For this review, take the finished solid that the model builds, in its own axes (mm). A direction names the side the tool comes from. Round coordinates to 2 decimals unless told otherwise and drop trailing zeros. Loops run counter-clockwise (first coordinate to the right, second up) from the corner with the lowest first, then second, coordinate; pieces in that order, holes last. Notation, with made-up numbers: M 36,-12 L 60,-12 A15 cw 60,8 Z; hole C -26,82.25 d5. An arc over 180 degrees is marked long. One line per question, with ' | ' between items. Start each with the question number.
1) Mouldability with a two-part tool opening along Z and no side actions: class faces 1 (the face through (-2.57, 0.8, -0.28)), 2 (the face through (4, 1, 0)), 3 (the face through (-1, 0, 1)) as pulls with the +Z half, pulls with the -Z half, needs draft (parallel to the pull), parting line crosses it, or undercut.
2) For probe 1 along X at (y, z) = (1.45, 1.75); probe 2 along X at (y, z) = (3.85, 4.5); probe 3 along Y at (x, z) = (-4.25, -5.5), list the stretches that pass through material, from the lowest coordinate up. Write a range as from..to.
3) For pin 1 Ø0.9 at (x, z) = (3.5, 3.5) entering from -Y; pin 2 Ø4 at (x, z) = (3, 6) entering from -Y; pin 3 Ø1 at (x, z) = (-3.97, 3.97) entering from -Y; pin 4 Ø0.9 at (x, y) = (3.5, 2) entering from -Z, all flat-tipped, find the tip position at first contact; note any pin that passes through.
4) For faces 4 (the face through (4.49, 2.53, 4.64)), 5 (the face through (-4, 1, -7.938)), 6 (the face through (3.862, 4.114, 6.405)), list the 3-axis set-ups (+Z, -Z, +X, -X, +Y, -Y) from which the entire face can be reached by the end or side of a thin tool; tool diameter is ignored.
5) We need section C-C (y = 3.9). Give the boundary of the cut face in (x, z).
```python
from build123d import *

# Parameters (mm, degrees)
SKETCH1_W               = 15.875
SKETCH1_H               = 15.875
BASE_EXTRUDE_DEPTH      = 3.175
SKETCH2_R               = 2.4384
BOSS_EXTRUDE1_DEPTH     = 1.905
LPATTERN4_COUNT         = 2
LPATTERN4_PITCH         = 7.9375
LPATTERN4_COUNT_DIR2    = 2
LPATTERN4_PITCH_DIR2    = 7.9375
CUT_EXTRUDE1_DEPTH      = 7.9375
CUT_EXTRUDE1_DEPTH_BACK = 12.6656949
SHELL1_T                = -1.5875
SKETCH4_R               = 1.27
BOSS_EXTRUDE2_DEPTH     = 1.5875
CUT_EXTRUDE2_START      = -1.5875
SKETCH5_R               = 0.635
CUT_EXTRUDE2_DEPTH      = 1.5875
FILLET1_R               = 0.254


with BuildPart() as part:
    # Sketch1 → Base-Extrude (new body)
    with BuildSketch(Plane(origin=(0, 0, 0), x_dir=(1, 0, 0), z_dir=(0, 1, 0))):
        Rectangle(SKETCH1_W, SKETCH1_H)
    extrude(amount=BASE_EXTRUDE_DEPTH)

    # Sketch2 → Boss-Extrude1 (add)
    with BuildSketch(Plane(origin=(0, 3.175, 0), x_dir=(-1, 0, 0), z_dir=(0, 1, 0))):
        with Locations(Location((3.96875, 3.96875, 0), (0, 0, 270))):
            Circle(SKETCH2_R)
    boss_extrude1 = extrude(amount=BOSS_EXTRUDE1_DEPTH)

    # LPattern4: Boss-Extrude1 2 × 2
    with Locations(*[(i * LPATTERN4_PITCH, 0, -j * LPATTERN4_PITCH_DIR2) for i in range(LPATTERN4_COUNT) for j in range(LPATTERN4_COUNT_DIR2) if (i, j) != (0, 0)]):
        add(boss_extrude1)

    # Sketch3 → Cut-Extrude1 (cut, two sides: drawn at the far end of the back side and taken through both)
    with BuildSketch(Plane(origin=(0, 3.175, 0), x_dir=(-1, 0, 0), z_dir=(0, 1, 0)).offset(-CUT_EXTRUDE1_DEPTH_BACK)):
        Polygon((0, -53.435079143), (0, -7.9375), (0, 0), (-7.9375, 0), (-53.435079143, 0), (-117.778372622, -64.343293479), (-64.343293479, -117.778372622), align=None)
    extrude(amount=CUT_EXTRUDE1_DEPTH + CUT_EXTRUDE1_DEPTH_BACK, mode=Mode.SUBTRACT)

    # Shell1
    shell1_openings = [part.faces().sort_by_distance(p)[0] for p in [
        (-1.322916667, 0, 1.322916667),
    ]]
    offset(amount=SHELL1_T, openings=shell1_openings, kind=Kind.INTERSECTION)

    # Sketch4 → Boss-Extrude2 (add)
    with BuildSketch(Plane.XZ.offset(-1.5875)):
        with Locations(Location((-3.81, 0, 0), (0, 0, 90))):
            Circle(SKETCH4_R)
        with Locations(Location((0, 3.81, 0), (0, 0, 90))):
            Circle(SKETCH4_R)
    extrude(amount=BOSS_EXTRUDE2_DEPTH)

    # Sketch5 → Cut-Extrude2 (cut)
    with BuildSketch(Plane.XZ.offset(CUT_EXTRUDE2_START)):
        with Locations(Location((0, 3.81, 0), (0, 0, 270))):
            Circle(SKETCH5_R)
        with Locations(Location((-3.81, 0, 0), (0, 0, 270))):
            Circle(SKETCH5_R)
    extrude(amount=CUT_EXTRUDE2_DEPTH, mode=Mode.SUBTRACT)

    # Fillet1
    fillet1_edges = [part.edges().sort_by_distance(p)[0] for p in [
        (7.9375, 3.175, 3.96875),
        (-3.96875, 3.175, -7.9375),
        (0, 3.175, -3.96875),
        (3.96875, 3.175, 0),
        (-7.9375, 3.175, 0),
        (0, 3.175, 7.9375),
    ]]
    fillet(fillet1_edges, radius=FILLET1_R)


solid = part.part
```
Answers below:
1) face 1: undercut | face 2: pulls with the -Z half | face 3: needs draft
2) probe 1: -7.94..-6.35, 6.35..7.94 | probe 2: -6.35..-1.59, 1.59..6.35 | probe 3: 1.59..5.08
3) pin 1: y = 1.59 | pin 2: y = 0 | pin 3: y = 3.49 | pin 4: z = 0
4) face 4: -Y | face 5: -Z, +X, -X, +Y, -Y | face 6: +Y
5) outline: C -3.97,-3.97 d4.88; C -3.97,3.97 d4.88; C 3.97,3.97 d4.88
